Here's how the part is built. I have some questions about the finished solid (model axes, mm). A direction names the side the tool comes from. Give positions to 0.01 mm unless a question says otherwise; leave off trailing zeros. Loops run counter-clockwise (first coordinate to the right, second up) from the corner with the lowest first, then second, coordinate; pieces in that order, holes last. Notation, with made-up numbers: (-3.75, -30) - (7.25, -30) arc R33 ccw to (7.25, 7) - close; hole circle Ø5 at (-29, -6). An arc over 180 degrees is marked (long way). Use one line per item in the form item = value.
Autodesk Inventor part; units mm, degrees
ref_plane "YZ Plane" through (0, 0, 0) normal (1, 0, 0) x (0, 1, 0)
ref_plane "XZ Plane" through (0, 0, 0) normal (0, 1, 0) x (-1, 0, 0)
ref_plane "XY Plane" through (0, 0, 0) normal (0, 0, 1) x (1, 0, 0)
sketch "Sketch1" plane through (0, 0, 0) normal (1, 0, 0) x (0, 1, 0)
  line L0 (0, 0) -> (12, 0)
  line L1 (12, 0) -> (12, -6.95)
  line L2 (12, -6.95) -> (0, -6.95)
  line L3 (0, -6.95) -> (0, 0)
  dimension "d0" = 12
  dimension "d1" = 6.95
extrude "Extrusion1" add sketch "Sketch1" along normal blind 0.3
sketch "Sketch2" plane through (0.3, 0, 0) normal (1, 0, 0) x (0, 0, -1)
  line L0 (0.975, 3.5) -> (5.975, 3.5)
  line L1 (5.975, 3.5) -> (5.975, 8.5)
  line L2 (5.975, 8.5) -> (0.975, 8.5)
  line L3 (0.975, 8.5) -> (0.975, 3.5)
  line L4 (6.95, 12) -> (0, 12)
  line L5 (6.95, 0) -> (6.95, 12)
  point P0 (0, 0)
  point P1 (3.475, 8.5)
  point P2 (3.475, 12)
  point P3 (5.975, 6)
  point P4 (6.95, 6)
  dimension "d4" = 5
  dimension "d5" = 5
extrude "Extrusion2" add sketch "Sketch2" along normal blind 1.5
sketch "Sketch3" plane through (1.8, 0, 0) normal (1, 0, 0) x (0, 0, -1)
  circle A0 centre (3.475, 6) radius 2
  line L0 (0.975, 3.5) -> (5.975, 3.5)
  line L1 (5.975, 3.5) -> (5.975, 8.5)
  point P0 (0, 0)
  point P1 (3.475, 3.5)
  point P2 (5.975, 6)
  dimension "d8" = 4
extrude "Extrusion3" cut sketch "Sketch3" against normal blind 0.2
chamfer "Chamfer1" distance 0.4 angle 45 1 edges at (1.05, 8.5, -5.975)
sketch "Sketch5" plane through (0.3, 0, 0) normal (1, 0, 0) x (0, 0, -1)
  line L0 (5.975, 3.5) -> (0.975, 3.5)
  line L1 (1.625, 3.5) -> (2.225, 3.5)
  line L2 (2.225, 3.5) -> (2.225, 2.9)
  line L3 (2.225, 2.9) -> (1.625, 2.9)
  line L4 (1.625, 2.9) -> (1.625, 3.5)
  line L5 (0.975, 3.5) -> (0.975, 8.5)
  line L6 (0.975, 6) -> (5.975, 6)
  line L7 (5.975, 8.1) -> (5.975, 3.5)
  line L8 (3.475, 3.5) -> (3.475, 8.5)
  line L9 (0.975, 8.5) -> (5.575, 8.5)
  line L10 (5.325, 3.5) -> (4.725, 3.5)
  line L11 (4.725, 3.5) -> (4.725, 2.9)
  line L12 (4.725, 2.9) -> (5.325, 2.9)
  line L13 (5.325, 2.9) -> (5.325, 3.5)
  line L14 (1.625, 8.5) -> (2.225, 8.5)
  line L15 (2.225, 8.5) -> (2.225, 9.1)
  line L16 (2.225, 9.1) -> (1.625, 9.1)
  line L17 (1.625, 9.1) -> (1.625, 8.5)
  line L18 (5.325, 8.5) -> (4.725, 8.5)
  line L19 (4.725, 8.5) -> (4.725, 9.1)
  line L20 (4.725, 9.1) -> (5.325, 9.1)
  line L21 (5.325, 9.1) -> (5.325, 8.5)
  point P0 (0, 0)
  dimension "d14" = 0.6
  dimension "d15" = 0.6
  dimension "d16" = 2.5
extrude "Extrusion4" add sketch "Sketch5" along normal blind 0.4 contours L19 L20 L21 L9 | L13 L12 L11 L0 | L2 L3 L4 L0 | L9 L17 L16 L15
sketch "Sketch6" plane through (0.3, 0, 0) normal (1, 0, 0) x (0, 0, -1)
  line L0 (2.375, 1.2) -> (4.575, 1.2)
  line L1 (4.575, 1.2) -> (4.575, 2.5)
  line L2 (4.575, 2.5) -> (2.375, 2.5)
  line L3 (2.375, 2.5) -> (2.375, 1.2)
  line L4 (0, 0) -> (6.95, 0)
  point P0 (3.475, 1.2)
  point P1 (3.475, 0)
  dimension "d20" = 2.2
  dimension "d21" = 1.2
  dimension "d24" = 2.5
extrude "Extrusion5" add sketch "Sketch6" along normal blind 1
properties part number "Base144"
(1) If we section it at B-B (y = 2.25): List the corners of the cut face in (x, z) for me (3 decimals).
Geometry says:
outline = (0, -6.95) - (0.3, -6.95) - (0.3, -4.575) - (1.3, -4.575) - (1.3, -2.375) - (0.3, -2.375) - (0.3, 0) - (0, 0) - close
(2) If I drill on probe 1 along Y at (x, z) = (1.05, -4); probe 2 along Y at (x, z) = (1.4, -5); probe 3 along X at (y, z) = (1.75, -5.5), over which ranges is the centre line in solid material (lowest first)?
Geometry says:
probe_1 = 1.2 to 2.5, 3.5 to 8.5
probe_2 = 3.5 to 8.5
probe_3 = 0 to 0.3
(3) If we section it at C-C (z = -2): List the corners of the cut face in (x, y) for me, plus the area to 3 significant figures.
Geometry says:
outline = (0, 0) - (0.3, 0) - (0.3, 2.9) - (0.7, 2.9) - (0.7, 3.5) - (1.8, 3.5) - (1.8, 4.65) - (1.6, 4.65) - (1.6, 7.35) - (1.8, 7.35) - (1.8, 8.5) - (0.7, 8.5) - (0.7, 9.1) - (0.3, 9.1) - (0.3, 12) - (0, 12) - close
area = 11.0 mm²
(4) Thinking about a two-plate mould opening in Z: for faces 5 (the flat face through (1, 2, -4.575)), 6 (the flat face through (1.6, 6, -3)), 7 (the flat face through (1, 2.5, -3)), which applies, pulls with the +Z half, pulls with the -Z half, needs draft (parallel to the pull), parting line crosses it, or undercut?
Geometry says:
face_5 = pulls with the -Z half
face_6 = undercut
face_7 = needs draft
(5) For faces 1 (the flat face through (1.3, 2, -3)), 2 (the flat face through (1, 6, -5.975)), 3 (the flat face through (1, 3.5, -3)), 4 (the flat face through (1, 2, -2.375)), which set-ups out of +Z, -Z, +X, -X, +Y, -Y let a thin tool reach every point of the face, with its end or its side?
Geometry says:
face_1 = +Z, -Z, +X, -Y
face_2 = -Z, +X, +Y, -Y
face_3 = +X
face_4 = +Z, +X, -Y
(6) If we section it at D-D (y = 5.25): List the corners of the cut face in (x, z) for me (3 decimals), plus the area to 3 significant figures.
Geometry says:
outline = (0, -6.95) - (0.3, -6.95) - (0.3, -5.975) - (1.8, -5.975) - (1.8, -5.329) - (1.6, -5.329) - (1.6, -1.621) - (1.8, -1.621) - (1.8, -0.975) - (0.3, -0.975) - (0.3, 0) - (0, 0) - close
area = 8.84 mm²
(7) If we section it at A-A (x = 0.95): List the corners of the cut face in (y, z) for me (3 decimals), plus the area to 3 significant figures.
Geometry says:
outline = (1.2, -4.575) - (2.5, -4.575) - (2.5, -2.375) - (1.2, -2.375) - close; (3.5, -5.975) - (8.1, -5.975) - (8.5, -5.575) - (8.5, -0.975) - (3.5, -0.975) - close
area = 27.8 mm²
(8) For P1, Ø0.7, axis at y = 9, z = -2, coming from the +X side, with a flat end and sliding along its axis, tell me the tip position at first contact or that it passes through.
Geometry says:
P1 = 0.7
